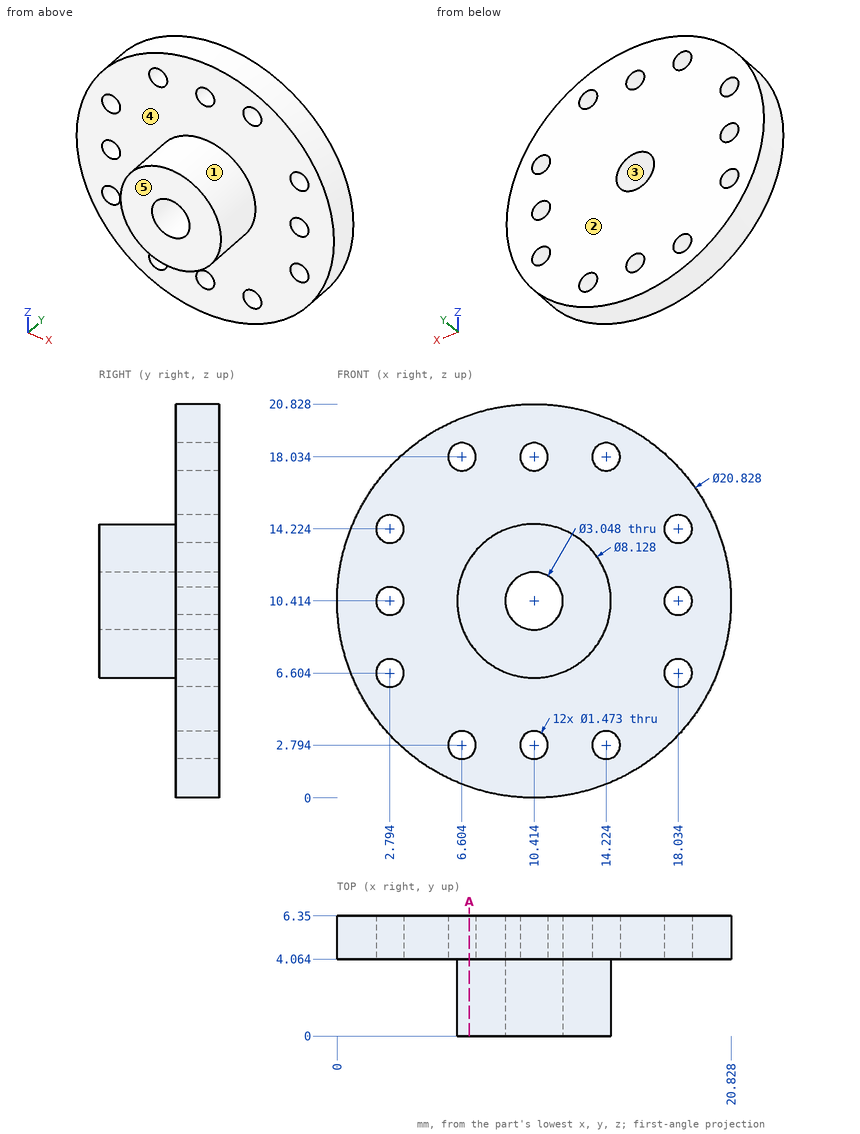
Study the drawing (mm; zero at the part's minimum x, y, z) and answer. A direction names the side the tool comes from. Round coordinates to 2 decimals unless told otherwise and drop trailing zeros.
1) Determine the mould class of the marked faces 1, 2 and 3 for opening direction Z: pulls with the +Z half, pulls with the -Z half, needs draft (parallel to the pull), parting line crosses it, or undercut.
2) Flat-ended cylindrical pins translate along their axes: P1, Ø2, axis at x = 6, y = 1, coming from the -Z side; P2, Ø2, axis at x = 6, y = 3.5, coming from the -Z side; P3, Ø3, axis at y = 4.5, z = 16.5, coming from the +X side. Find the tip coordinate at first contact, or state that the pin passes through.
3) Which of the six approach directions +Z, -Z, +X, -X, +Y, -Y give full straight-line access (tool end or side, diameter ignored) to the marked faces 4 and 5?
4) A cutting plane is placed at A-A on x = 7. Give the number of separate pieces and of enclosed holes in the cut face, and give its area (3 significant figures).
5) Consider probe 1 along Z at (x, y) = (6.5, 5) (1 decimal); probe 2 along X at (y, z) = (6.25, 7) (1 decimal); probe 3 along X at (y, z) = (5.5, 9.75) (1 decimal). Determine where each line is inside the solid, lowest interval first.
Entries:
1. face 1: parting line crosses it
1. face 2: needs draft
1. face 3: undercut
2. P1: stops at z = 8.21
2. P2: stops at z = 0.64
2. P3: stops at x = 19.76
3. face 4: -Y
3. face 5: +Z, -Z, +X, -X, -Y
4. separate pieces: 3
4. enclosed holes: 0
4. area: 57.2 mm2
5. probe 1: z = 0.8 to 2.1, 3.5 to 17.3, 18.8 to 20.1
5. probe 2: x = 0.6 to 2.2, 3.4 to 17.4, 18.7 to 20.3
5. probe 3: x = 0 to 2.5, 3.1 to 9, 11.8 to 17.7, 18.4 to 20.8
